from build123d import *

# Parameters (mm, degrees)
SKETCH080_W             = 110
SKETCH080_H             = 110
PAD051_DEPTH            = 220
POCKET036_DEPTH         = 158
POCKET037_DEPTH         = 158
THICKNESS002_T          = 6
SKETCH079_W             = 5
SKETCH079_H             = 5
PAD052_DEPTH            = 110
BODY012_PLACEMENT_ANGLE = 90


with BuildPart() as part:
    # Sketch080 → Pad051 (new body)
    with BuildSketch(Plane.XY):
        Rectangle(SKETCH080_W, SKETCH080_H)
    extrude(amount=PAD051_DEPTH)

    # Sketch081 (on Face3 of Pad051) → Pocket036 (cut)
    with BuildSketch(Plane.XZ.offset(55)):
        Polygon((-55, 20), (-30.5, 200), (-30.5, 220), (-55, 220), align=None)
        Polygon((30.5, 220), (55, 220), (55, 20), (30.5, 200), align=None)
    extrude(amount=-POCKET036_DEPTH, mode=Mode.SUBTRACT)

    # Sketch082 (on DatumPlane) → Pocket037 (cut)
    with BuildSketch(Plane.YZ.offset(55)):
        Polygon((-55, 20), (-22, 200), (-22, 220), (-55, 220), align=None)
        Polygon((22, 220), (22, 200), (55, 20), (55, 220), align=None)
    extrude(amount=-POCKET037_DEPTH, mode=Mode.SUBTRACT)

    # Thickness002
    thickness002_openings = [part.faces().sort_by_distance(p)[0] for p in [
        (0, 0, 220),
    ]]
    offset(amount=THICKNESS002_T, openings=thickness002_openings)

    # Sketch079 → Pad052 (join)
    with BuildSketch(Plane(origin=(0, -55, 0), x_dir=(-1, 0, 0), z_dir=(0, 1, 0))):
        with Locations((-52.5, 6.5)):
            Rectangle(SKETCH079_W, SKETCH079_H)
        with Locations((52.5, 6.5)):
            Rectangle(SKETCH079_W, SKETCH079_H)
    extrude(amount=PAD052_DEPTH)


with BuildPart() as part_1:
    # Body012 placement: moved
    add(part.part.moved(Location((-0.100429, -201, -6.066442))).rotate(Axis((-0.100429, -201, -6.066442), (-1, 0, 0)), BODY012_PLACEMENT_ANGLE))


solid = part_1.part
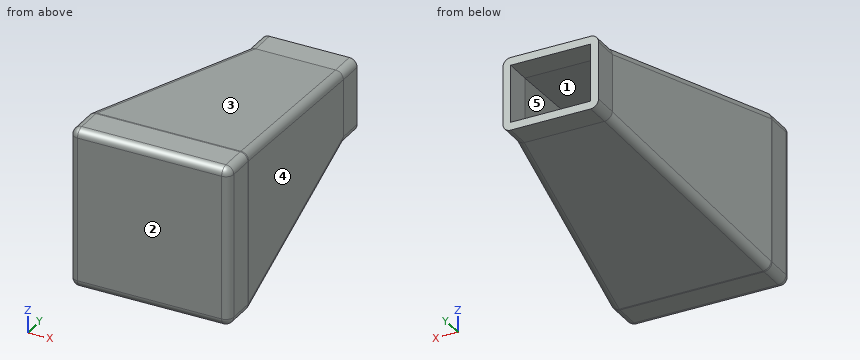
The listing builds one solid part. Answer for the finished solid, in the listing's coordinates (mm). Face numbers are marked on the shaded views. A direction names the side the tool comes from. Coordinates: 2 decimals unless noted, no trailing zeros. Order: outer loops, then holes, each group sorted by start corner. A loop starts at its lowest first (then second) coordinate and runs counter-clockwise, first axis right, second up.
Q1. A cutting plane is placed at B-B, the plane z = -2. Write down the section's boundary in (x, y).
Q2. Which of the six approach directions +Z, -Z, +X, -X, +Y, -Y give full straight-line access (tool end or side, diameter ignored) to the marked faces 4 and 5?
Q3. A cutting plane is placed at A-A, the plane x = 3. Write down the section's boundary in (y, z), and give its area (3 significant figures).
Q4. Consider line 1 (Z direction, x = 34, y = -177.5); line 2 (X direction, y = -69.5, z = -10); line 3 (Z direction, x = 40, y = -78.5). Determine where each line is inside the solid, lowest interval first.
Q5. Given P1, Ø5, axis at y = -174.5, z = -5, coming from the +X side; P2, Ø5, axis at y = -164, z = -50, coming from the -X side; P3, Ø5, axis at x = 11.5, y = -163.5, coming from the +Z side, each flat-ended and moving along its own axis, determine where each tip first touches the part or whether it passes through.
Q6. For a pull along Y with two mould halves and no side action, classify the marked faces 1, 2 and 3 as pulls with the +Y half, pulls with the -Y half, needs draft (parallel to the pull), parting line crosses it, or undercut.
Answers follow:
1. outline: (-61.1, -201) arc R6 ccw to (-55.1, -207) - (54.9, -207) arc R6 ccw to (60.9, -201) - (60.9, -181) arc R6 ccw to (60.84, -180.19) - (36.4, -0.59) - (36.4, 19) - (30.4, 19) - (30.4, -1) - (54.9, -181) - (54.9, -192) - (49.9, -192) - (49.9, -197) - (54.9, -197) - (54.9, -201) - (-55.1, -201) - (-55.1, -197) - (-50.1, -197) - (-50.1, -192) - (-55.1, -192) - (-55.1, -181) - (-30.6, -1) - (-30.6, 19) - (-36.6, 19) - (-36.6, -0.59) - (-61.05, -180.19) arc R6 ccw to (-61.1, -181) - close
2. face 4: +Z, -Z, +X, +Y
2. face 5: none
3. outline: (-207, -61.07) arc R6 ccw to (-201, -67.07) - (-181, -67.07) arc R6 ccw to (-179.92, -66.97) - (-0.45, -34.07) - (19, -34.07) - (19, -28.07) - (-1, -28.07) - (-181, -61.07) - (-201, -61.07) - (-201, 48.93) - (-181, 48.93) - (-1, 15.93) - (19, 15.93) - (19, 21.93) - (-0.45, 21.93) - (-179.92, 54.84) arc R6 ccw to (-181, 54.93) - (-201, 54.93) arc R6 ccw to (-207, 48.93) - close
3. area: 3,390 mm2
4. line 1: z = -66.52 to -60.42, 48.29 to 54.39
4. line 2: x = -45.98 to -39.92, 39.72 to 45.78
4. line 3: z = -48.37 to -42.27, 30.14 to 36.24
5. P1: stops at x = 60.41
5. P2: stops at x = -59.18
5. P3: stops at z = 52.28
6. face 1: undercut
6. face 2: pulls with the -Y half
6. face 3: pulls with the +Y half
